Verification items for the finished model (mm, model axes). A direction names the side the tool comes from. Give positions to 0.01 mm unless a question says otherwise; leave off trailing zeros. Order: outer loops, then holes, each group sorted by start corner. A loop starts at its lowest first (then second) coordinate and runs counter-clockwise, first axis right, second up. Notation, with made-up numbers: (-16.5, 39) - (13.5, 39) arc R17 ccw to (13.5, 70) - close; hole circle Ø2 at (-3, 10). An arc over 180 degrees is marked (long way). Answer as a JSON object with one key per item and string values.
```python
from build123d import *

# Parameters (mm, degrees)
STOCK_SPINE_MASTER_1_START     = -18.2
STOCK_SPINE_MASTER_1_OUTLINE_W = 39
STOCK_SPINE_MASTER_1_OUTLINE_H = 97.215728753
STOCK_SPINE_MASTER_1_OUTLINE_R = 2.25
STOCK_SPINE_MASTER_1_DEPTH     = 3.2
FILLET2_R                      = 5
CUT_EXTRUDE1_DEPTH             = 174.131424069
FILLET5_R                      = 2


# Read off the part's stored shape, not the designer's step: Stock-spine_master-1
with BuildPart() as part:
    # Stock-spine_master-1 outline → Stock-spine_master-1 (new body)
    with BuildSketch(Plane.XY.offset(STOCK_SPINE_MASTER_1_START)):
        with Locations((0, -123.392135623)):
            Rectangle(STOCK_SPINE_MASTER_1_OUTLINE_W, STOCK_SPINE_MASTER_1_OUTLINE_H)
        with Locations((0, -139.392135624)):
            Circle(STOCK_SPINE_MASTER_1_OUTLINE_R, mode=Mode.SUBTRACT)
        with Locations((0, -107.392135624)):
            Circle(STOCK_SPINE_MASTER_1_OUTLINE_R, mode=Mode.SUBTRACT)
    extrude(amount=STOCK_SPINE_MASTER_1_DEPTH)

    # Fillet2
    fillet2_edges = [part.edges().sort_by_distance(p)[0] for p in [
        (19.5, -172, -16.6),
        (19.5, -74.784271247, -16.6),
        (-19.5, -74.784271247, -16.6),
        (-19.5, -172, -16.6),
    ]]
    fillet(fillet2_edges, radius=FILLET2_R)

    # Sketch1 → Cut-Extrude1 (cut, through all)
    with BuildSketch(Plane.XY.offset(-15)):
        with BuildLine():
            Line((-6.248354978, -107.24874781), (-13.5, -103.062008605))
            Line((-13.5, -103.062008605), (-13.5, -143.722262643))
            Line((-13.5, -143.722262643), (-6.248354978, -139.535523437))
            ThreePointArc((-6.248354978, -139.535523437), (-6.249588731, -139.463834249), (-6.25, -139.392135624))
            Line((-6.25, -139.392135624), (-6.25, -107.392135624))
            ThreePointArc((-6.25, -107.392135624), (-6.249588731, -107.320436999), (-6.248354978, -107.24874781))
        make_face()
        with BuildLine():
            Line((13.5, -80.784271247), (-13.5, -80.784271247))
            Line((-13.5, -80.784271247), (-13.5, -96.133805375))
            Line((-13.5, -96.133805375), (-3.248354978, -102.052595387))
            ThreePointArc((-3.248354978, -102.052595387), (0, -101.142135624), (3.248354978, -102.052595387))
            Line((3.248354978, -102.052595387), (13.5, -96.133805375))
            Line((13.5, -96.133805375), (13.5, -80.784271247))
        make_face()
        with BuildLine():
            Line((13.5, -143.722262643), (13.5, -103.062008605))
            Line((13.5, -103.062008605), (6.248354978, -107.24874781))
            ThreePointArc((6.248354978, -107.24874781), (6.249588731, -107.320436999), (6.25, -107.392135624))
            Line((6.25, -107.392135624), (6.25, -139.392135624))
            ThreePointArc((6.25, -139.392135624), (6.249588731, -139.463834249), (6.248354978, -139.535523437))
            Line((6.248354978, -139.535523437), (13.5, -143.722262643))
        make_face()
        with BuildLine():
            Line((-3.248354978, -144.73167586), (-13.5, -150.650465873))
            Line((-13.5, -150.650465873), (-13.5, -166))
            Line((-13.5, -166), (13.5, -166))
            Line((13.5, -166), (13.5, -150.650465873))
            Line((13.5, -150.650465873), (3.248354978, -144.73167586))
            ThreePointArc((3.248354978, -144.73167586), (0, -145.642135624), (-3.248354978, -144.73167586))
        make_face()
    extrude(amount=-CUT_EXTRUDE1_DEPTH, mode=Mode.SUBTRACT)

    # Fillet5
    # the kernel refuses this fillet: 2 mm, written as the material it adds along each edge
    with BuildSketch(Plane(origin=(-6.248354978, -107.24874781, -15), x_dir=(-0.8660254037844632, 0.4999999999999575, 0), z_dir=(0, 0, -1)), Plane(origin=(6.248354978, -139.535523437, -15), x_dir=(0.8660254037844526, -0.4999999999999759, 0), z_dir=(0, 0, -1))) as fillet5_piece_1:
        with BuildLine():
            CenterArc((1.156600046, -2), FILLET5_R, 90, 60)
            Line((-0.575450762, -1), (-0.748655843, -0.9))
            ThreePointArc((-0.748655843, -0.9), (-0.243474357, -0.025), (-0.175453698, 0.096))
            Line((-0.175453698, 0.096), (0, 0.2))
            Line((0, 0.2), (1.156600046, 0.2))
            Line((1.156600046, 0.2), (1.156600046, 0))
        make_face()
    extrude(amount=3.2)
    with BuildSketch(Plane(origin=(6.248354978, -107.24874781, -15), x_dir=(0.8660254037844632, 0.4999999999999575, 0), z_dir=(0, 0, -1)), Plane(origin=(-6.248354978, -139.535523437, -15), x_dir=(-0.8660254037844523, -0.4999999999999766, 0), z_dir=(0, 0, -1))) as fillet5_piece_2:
        with BuildLine():
            CenterArc((1.156600046, 2), FILLET5_R, 210, 60)
            Line((-0.575450762, 1), (-0.748655843, 0.9))
            ThreePointArc((-0.748655843, 0.9), (-0.243474357, 0.025), (-0.175453698, -0.096))
            Line((-0.175453698, -0.096), (0, -0.2))
            Line((0, -0.2), (1.156600046, -0.2))
            Line((1.156600046, -0.2), (1.156600046, 0))
        make_face()
    extrude(amount=3.2)
    with BuildSketch(Plane(origin=(-13.5, -166, -15), x_dir=(0, 1, 0), z_dir=(0, 0, -1)), Plane(origin=(13.5, -166, -15), x_dir=(-1, 0, 0), z_dir=(0, 0, -1)), Plane(origin=(-13.5, -80.784271247, -15), x_dir=(1, 0, 0), z_dir=(0, 0, -1))) as fillet5_piece_3:
        with BuildLine():
            CenterArc((FILLET5_R, FILLET5_R), FILLET5_R, 180, 90)
            Line((0, FILLET5_R), (0, 0))
            Line((0, 0), (FILLET5_R, 0))
        make_face()
    extrude(amount=3.2)
    with BuildSketch(Plane(origin=(13.5, -150.650465873, -15), x_dir=(0, -1, 0), z_dir=(0, 0, -1)), Plane(origin=(13.5, -96.133805375, -15), x_dir=(-0.8660254037844395, -0.49999999999999867, 0), z_dir=(0, 0, -1)), Plane(origin=(-13.5, -96.133805375, -15), x_dir=(0, 1, 0), z_dir=(0, 0, -1)), Plane(origin=(-13.5, -150.650465873, -15), x_dir=(0.8660254037844375, 0.5000000000000019, 0), z_dir=(0, 0, -1))) as fillet5_piece_4:
        with BuildLine():
            CenterArc((FILLET5_R * 0.57735026919, FILLET5_R), FILLET5_R, 210, 60)
            Line((-FILLET5_R * 0.288675134595, FILLET5_R * 0.5), (0, 0))
            Line((0, 0), (FILLET5_R * 0.57735026919, 0))
        make_face()
    extrude(amount=3.2)
    with BuildSketch(Plane(origin=(13.5, -143.722262643, -15), x_dir=(-0.8660254037844394, 0.4999999999999986, 0), z_dir=(0, 0, -1)), Plane(origin=(13.5, -103.062008605, -15), x_dir=(0, -1, 0), z_dir=(0, 0, -1)), Plane(origin=(-13.5, -103.062008605, -15), x_dir=(0.866025403784438, -0.500000000000001, 0), z_dir=(0, 0, -1)), Plane(origin=(-13.5, -143.722262643, -15), x_dir=(0, 1, 0), z_dir=(0, 0, -1))) as fillet5_piece_5:
        with BuildLine():
            CenterArc((FILLET5_R * 1.73205080757, FILLET5_R), FILLET5_R, 150, 120)
            Line((FILLET5_R * 0.866025403784, FILLET5_R * 1.5), (0, 0))
            Line((0, 0), (FILLET5_R * 1.73205080757, 0))
        make_face()
    extrude(amount=3.2)
    with BuildSketch(Plane(origin=(13.5, -80.784271247, -15), x_dir=(-1, 0, 0), z_dir=(0, 0, -1))) as fillet5_piece_6:
        with BuildLine():
            CenterArc((FILLET5_R, -FILLET5_R), FILLET5_R, 90, 90)
            Line((0, -FILLET5_R), (0, 0))
            Line((0, 0), (FILLET5_R, 0))
        make_face()
    extrude(amount=3.2)
    with BuildSketch(Plane(origin=(3.248354978, -144.73167586, -15), x_dir=(0.866025403784452, -0.49999999999997674, 0), z_dir=(0, 0, -1)), Plane(origin=(-3.248354978, -102.052595387, -15), x_dir=(-0.8660254037844742, 0.4999999999999385, 0), z_dir=(0, 0, -1))) as fillet5_piece_7:
        with BuildLine():
            CenterArc((1.079274324, 2), FILLET5_R, 217.305200966, 52.694799034)
            ThreePointArc((-0.511562615, 0.787878788), (-0.240957875, 0.403564115), (0, 0))
            Line((0, 0), (1.079274324, 0))
        make_face()
    extrude(amount=3.2)
    with BuildSketch(Plane(origin=(-3.248354978, -144.73167586, -15), x_dir=(-0.8660254037844329, -0.5000000000000099, 0), z_dir=(0, 0, -1))) as fillet5_piece_8:
        with BuildLine():
            CenterArc((1.079274324, -2), FILLET5_R, 90, 52.694799034)
            ThreePointArc((-0.511562615, -0.787878788), (-0.240957875, -0.403564115), (0, 0))
            Line((0, 0), (1.079274324, 0))
        make_face()
    extrude(amount=3.2)
    with BuildSketch(Plane(origin=(3.248354978, -102.052595387, -15), x_dir=(-0.8909692919420457, 0.4540635647310734, 0), z_dir=(0, 0, -1))) as fillet5_piece_9:
        with BuildLine():
            CenterArc((1.089689758, 1.994344328), FILLET5_R, 212.99530149, 52.694799034)
            Line((-0.587740698, 0.905203811), (0, 0))
            ThreePointArc((0, 0), (0.469693861, 0.017673975), (0.939387723, 0))
        make_face()
    extrude(amount=3.2)


solid = part.part
```
(1) Release check for a two-part mould opening along X. For faces 1 (the cylindrical face through (-6.525, -107.39, -16.578)), 2 (the flat face through (0, -123, -15)), 3 (the cylindrical face through (6.51, -107.42, -16.58)), 4 (the cylindrical face through (-18.074, -76.288, -16.578)) record: pulls with the +X half, pulls with the -X half, needs draft (parallel to the pull), parting line crosses it, or undercut.
Computed values:
{"face 1": "undercut", "face 2": "needs draft", "face 3": "undercut", "face 4": "pulls with the -X half"}
(2) Gauge pin test, flat end, axial feed: pin 1 Ø8 at (x, y) = (10, -97) entering from -Z. Record the tip position at first contact, or that the pin passes through.
Computed values:
{"pin 1": "stops at z = -18.2"}
(3) Section check A-A (y = -157.5). Record the cut outline in (x, z).
Computed values:
{"outline": "(-19.5, -18.2) - (-13.5, -18.2) - (-13.5, -15) - (-19.5, -15) - close; (13.5, -18.2) - (19.5, -18.2) - (19.5, -15) - (13.5, -15) - close"}
(4) Access from +Z, -Z, +X, -X, +Y, -Y to the whole of each face (thin tool, end or side, straight path). Record for faces 5 (the flat face through (0, -172, -17)), 6 (the flat face through (-8.4, -99.08, -16.58)).
Computed values:
{"face 5": "+Z, -Z, +X, -X, -Y", "face 6": "+Z, -Z"}
(5) Material ranges on line 1 along X through (y, z) = (-118.5, -16.3); line 2 along Y through (x, z) = (0, -17.1); line 3 along X through (y, z) = (-82.5, -17.1), recorded low to high. Write a range as [from, to].
Computed values:
{"line 1": "x = [-19.5, -13.5], [-6.25, 6.25], [13.5, 19.5]", "line 2": "y = [-172, -166], [-145.64, -141.64], [-137.14, -109.64], [-105.14, -101.14], [-80.78, -74.78]", "line 3": "x = [-19.5, -13.48], [13.48, 19.5]"}
(6) Section check C-C (z = -15.8). Count the separate pieces of the cut face and the enclosed holes in it, then the cut area to 3 significant figures.
Computed values:
{"separate pieces": "1", "enclosed holes": "6", "area": "2,210 mm²"}
(7) Section check B-B (x = 0). Record the cut outline in (y, z).
Computed values:
{"outline": "(-172, -18.2) - (-166, -18.2) - (-166, -15) - (-172, -15) - close; (-145.64, -18.2) - (-141.64, -18.2) - (-141.64, -15) - (-145.64, -15) - close; (-137.14, -18.2) - (-109.64, -18.2) - (-109.64, -15) - (-137.14, -15) - close; (-105.14, -18.2) - (-101.14, -18.2) - (-101.14, -15) - (-105.14, -15) - close; (-80.78, -18.2) - (-74.78, -18.2) - (-74.78, -15) - (-80.78, -15) - close"}
